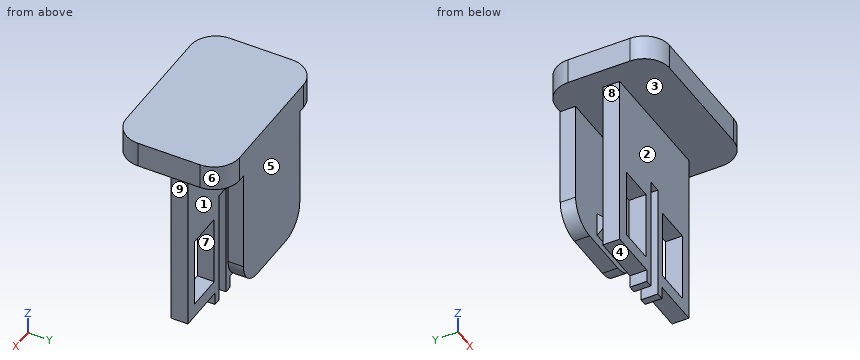
from build123d import *

# Parameters (mm, degrees)
F1_DEPTH = 5
F3_DEPTH = 3
F5_DEPTH = 2.35
F7_W     = 7
F7_H     = 13.75
F8_DEPTH = 3.3


with BuildPart() as f1:
    # F0 (on Top) → F1 (new body)
    with BuildSketch(Plane.XY):
        with BuildLine():
            ThreePointArc((16.33, 6.075), (14.8655339059, 9.6105339059), (11.33, 11.075))
            Line((11.33, 11.075), (-11.33, 11.075))
            ThreePointArc((-11.33, 11.075), (-14.8655339059, 9.6105339059), (-16.33, 6.075))
            Line((-16.33, 6.075), (-16.33, -6.075))
            ThreePointArc((-16.33, -6.075), (-14.8655339059, -9.6105339059), (-11.33, -11.075))
            Line((-11.33, -11.075), (11.33, -11.075))
            ThreePointArc((11.33, -11.075), (14.8655339059, -9.6105339059), (16.33, -6.075))
            Line((16.33, -6.075), (16.33, 6.075))
        make_face()
    extrude(amount=F1_DEPTH)

    # F2 (on face) → F3 (join)
    with BuildSketch(Plane(origin=(0, 11.075, 0), x_dir=(-1, 0, 0), z_dir=(0, 1, 0))):
        with BuildLine():
            Line((10, -20), (10, 5))
            Line((10, 5), (-10, 5))
            Line((-10, 5), (-10, -20))
            ThreePointArc((-10, -20), (-8.5355339059, -23.5355339059), (-5, -25))
            Line((-5, -25), (5, -25))
            ThreePointArc((5, -25), (8.5355339059, -23.5355339059), (10, -20))
        make_face()
    extrude(amount=-F3_DEPTH)

    # F4 (on Right) → F5 (join, symmetric)
    with BuildSketch(Plane.YZ):
        Polygon((5.575, -20.645), (8.075, -23), (8.075, -18.29), align=None)
    extrude(amount=F5_DEPTH, both=True)

    # F7 (on offset) → F8 (join)
    with BuildSketch(Plane.XZ.offset(-1.475)):
        Polygon((12.3, 5), (-12.3, 5), (-12.3, -34.75), (-2.68, -34.75), (-2.68, -37.25), (-1.25, -37.25), (-1.25, -14.34), (1.25, -14.34), (1.25, -37.25), (2.68, -37.25), (2.68, -34.75), (12.3, -34.75), align=None)
        with Locations((-6.45, -25.175)):
            Rectangle(F7_W, F7_H, mode=Mode.SUBTRACT)
        with Locations((6.45, -25.175)):
            Rectangle(F7_W, F7_H, mode=Mode.SUBTRACT)
    extrude(amount=F8_DEPTH)


solid = f1.part
The listing builds one solid part. Answer for the finished solid, in the listing's coordinates (mm). Face numbers are marked on the shaded views. A direction names the side the tool comes from. Round coordinates to 2 decimals unless told otherwise and drop trailing zeros. Order: outer loops, then holes, each group sorted by start corner. A loop starts at its lowest first (then second) coordinate and runs counter-clockwise, first axis right, second up. Notation, with made-up numbers: (-34, 59) -> (-14, 59) arc R32 ccw to (-14, 89) -> close; hole circle Ø10 at (38.5, 89). An arc over 180 degrees is marked (long way). Write each question's results on one line, items separated by ' | '. Start each with the question number.
Q1. Each of these flat-tipped pins is pushed along its axis until it touches: pin 1 (3.5 mm diameter, centred on y = 0, z = -23, fed in from -X); pin 2 (1.5 mm diameter, centred on x = -9, z = -9, fed in from -Y) (3 decimals); pin 3 (11 mm diameter, centred on x = -1, y = 2.5, fed in from -Z); pin 4 (12 mm diameter, centred on x = -5, y = -9, fed in from -Z). Where does it stop, or does it pass through?
Q2. The mould has two halves that part along Y. Classify the marked faces 1, 2, 3 and 4: pulls with the +Y half, pulls with the -Y half, needs draft (parallel to the pull), parting line crosses it, or undercut.
Q3. Find section B-B (x = -9). Determine the outline of the cut face in (y, z) (3 decimals), then the cut area to 3 significant figures.
Q4. Find section C-C (z = -16.5). Determine the outline of the cut face in (x, y) (3 decimals).
Q5. Find section A-A (z = -34). Determine the outline of the cut face in (x, y) (3 decimals).
Q6. Straight lines are drawn through the part: probe 1 along X at (y, z) = (0.5, -19); probe 2 along Y at (x, z) = (6, -9) (3 decimals); probe 3 along Z at (x, y) = (-14, -6.5). For each, find the intervals that lie inside material, in ascending order. Write a range as from..to.
Q7. Find section D-D (x = -4.5). Determine the outline of the cut face in (y, z) (3 decimals).
Q8. Which of the six approach directions +Z, -Z, +X, -X, +Y, -Y give full straight-line access (tool end or side, diameter ignored) to the marked faces 5, 6, 7, 8 and 9?
Worked answers:
1) pin 1: stops at x = -12.3 | pin 2: stops at y = -1.825 | pin 3: stops at z = -37.25 | pin 4: stops at z = 0
2) face 1: undercut | face 2: pulls with the -Y half | face 3: undercut | face 4: needs draft
3) outline: (-11.075, 0) -> (-1.825, 0) -> (-1.825, -18.3) -> (1.475, -18.3) -> (1.475, 0) -> (8.075, 0) -> (8.075, -23) -> (11.075, -23) -> (11.075, 5) -> (-11.075, 5) -> close; (-1.825, -34.75) -> (1.475, -34.75) -> (1.475, -32.05) -> (-1.825, -32.05) -> close | area: 249 mm2
4) outline: (-12.3, -1.825) -> (-1.25, -1.825) -> (-1.25, 1.475) -> (-12.3, 1.475) -> close; (-10, 8.075) -> (10, 8.075) -> (10, 11.075) -> (-10, 11.075) -> close; (1.25, -1.825) -> (12.3, -1.825) -> (12.3, 1.475) -> (1.25, 1.475) -> close
5) outline: (-12.3, -1.825) -> (-1.25, -1.825) -> (-1.25, 1.475) -> (-12.3, 1.475) -> close; (1.25, -1.825) -> (12.3, -1.825) -> (12.3, 1.475) -> (1.25, 1.475) -> close
6) probe 1: x = -12.3..-9.95, -2.95..-1.25, 1.25..2.95, 9.95..12.3 | probe 2: y = -1.825..1.475, 8.075..11.075 | probe 3: z = 0..5
7) outline: (-11.075, 0) -> (-1.825, 0) -> (-1.825, -18.3) -> (1.475, -18.3) -> (1.475, 0) -> (8.075, 0) -> (8.075, -25) -> (11.075, -25) -> (11.075, 5) -> (-11.075, 5) -> close; (-1.825, -34.75) -> (1.475, -34.75) -> (1.475, -32.05) -> (-1.825, -32.05) -> close
8) face 5: +Z, -Z, +X, -X, +Y | face 6: +Z, -Z, +X, +Y | face 7: -Y | face 8: -Z, -X, +Y, -Y | face 9: -Z, +X, +Y, -Y
